Input: dimensioned drawing with shaded views. Units: mm. Origin: part minimum x, y, z. A direction names the side the tool comes from. Round coordinates to 2 decimals unless told otherwise and drop trailing zeros. Loops run counter-clockwise (first coordinate to the right, second up) from the corner with the lowest first, then second, coordinate; pieces in that order, holes last. Notation, with made-up numbers: (-27, -31.75) - (-14, -31.75) arc R14 cw to (-14, -18.75) - close; hole circle Ø11 at (-27.75, -9.75). An arc over 180 degrees is marked (long way). Answer as a JSON object with one key per item and string values. Group by question number.
Item 1: Line query: line 1 (Z direction, x = 74, y = 283); line 2 (Z direction, x = 115, y = 4); line 3 (X direction, y = 2.5, z = 165). Output: solid intervals per line, ascending.
Item 2: Reachability of the marked faces 1, 2 and 3 from +Z, -Z, +X, -X, +Y, -Y: full face, straight path, thin tool, end or side. Return the list, or none.
Item 3: Section B-B (z = 110). Return the cut outline in (x, y), plus the area to 3 significant figures.
Item 4: Section C-C (x = 115). Return the cut outline in (y, z).
Item 5: First-contact query: pin 1 (4 mm diameter, centred on y = 208, z = 84.5, fed in from +X); pin 2 (12 mm diameter, centred on x = 115, z = 165, fed in from +Y); pin 3 (3 mm diameter, centred on x = 40.5, z = 102, fed in from +Y); pin 4 (9.5 mm diameter, centred on y = 283, z = 195, fed in from -X). Flat tips, straight axial feed; report the tip coordinate or a pass-through.
Item 6: Section A-A (y = 198). Return the cut outline in (x, z), plus the area to 3 significant figures.
Item 7: Section D-D (z = 138). Return the cut outline in (x, y).
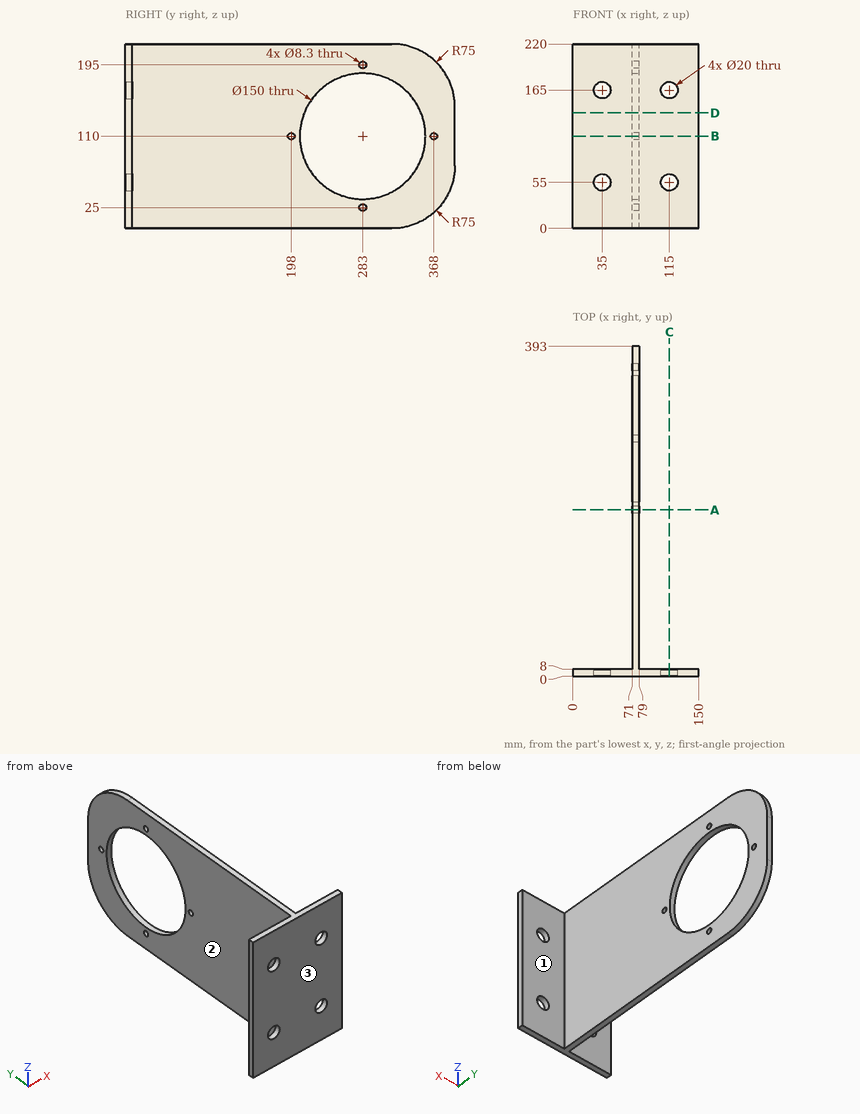
Values:
{
 "1": {"line 1": "z = 0 to 20.85, 29.15 to 35, 185 to 190.85, 199.15 to 220", "line 2": "z = 0 to 45, 65 to 155, 175 to 220", "line 3": "x = 0 to 25, 45 to 105, 125 to 150"},
 "2": {"face 1": "+Z, -Z, +X, +Y", "face 2": "+Z, -Z, -X, +Y", "face 3": "+Z, -Z, +X, -X, -Y"},
 "3": {"outline": "(0, 0) - (150, 0) - (150, 8) - (79, 8) - (79, 193.85) - (71, 193.85) - (71, 8) - (0, 8) - close; (71, 202.15) - (79, 202.15) - (79, 208) - (71, 208) - close; (71, 358) - (79, 358) - (79, 363.85) - (71, 363.85) - close; (71, 372.15) - (79, 372.15) - (79, 393) - (71, 393) - close", "area": "2,950 mm^2"},
 "4": {"outline": "(0, 0) - (8, 0) - (8, 45) - (0, 45) - close; (0, 65) - (8, 65) - (8, 155) - (0, 155) - close; (0, 175) - (8, 175) - (8, 220) - (0, 220) - close"},
 "5": {"pin 1": "stops at x = 79", "pin 2": "passes through", "pin 3": "stops at y = 8", "pin 4": "stops at x = 71"},
 "6": {"outline": "(71, 0) - (79, 0) - (79, 105.85) - (71, 105.85) - close; (71, 114.15) - (79, 114.15) - (79, 220) - (71, 220) - close", "area": "1,690 mm^2"},
 "7": {"outline": "(0, 0) - (150, 0) - (150, 8) - (79, 8) - (79, 213.42) - (71, 213.42) - (71, 8) - (0, 8) - close; (71, 352.58) - (79, 352.58) - (79, 393) - (71, 393) - close"}
}
